```python
from build123d import *

# Parameters (mm, degrees)
SKETCH_1_W                 = 40
SKETCH_1_H                 = 20
EXTRUDE_1_DEPTH            = 28.5
SKETCH_7_R                 = 2.5
EXTRUDE_4_DEPTH            = 6.975384219
SKETCH_1_2_W               = 40
SKETCH_1_2_H               = 20
EXTRUDE_5_DEPTH            = 7.5
SKETCH_3_W                 = 53
SKETCH_3_H                 = 18
EXTRUDE_6_DEPTH            = 2
CUT_EXTRUDE_4_DEPTH        = 5
EXTRUDE_7_DEPTH            = 1.5
SKETCH_13_W                = 12
SKETCH_13_H                = 19
EXTRUDE_8_DEPTH            = 2
SKETCH_14_R                = 6
EXTRUDE_9_DEPTH            = 1.5
EXTRUDE_10_DEPTH           = 0.25
CUT_EXTRUDE_5_DEPTH        = 50
CUT_EXTRUDE_6_DEPTH        = 50
CUT_EXTRUDE_11_DEPTH       = 1.2
SKETCH_25_R                = 1.5
EXTRUDE_12_DEPTH           = 1
EXTRUDE_12_DRAFT           = 15
EXTRUDE_12_PROFILE_2_DEPTH = 1
EXTRUDE_12_PROFILE_2_DRAFT = 15
EXTRUDE_12_PROFILE_3_DEPTH = 1
EXTRUDE_12_PROFILE_3_DRAFT = 15
EXTRUDE_12_PROFILE_4_DEPTH = 1
EXTRUDE_12_PROFILE_4_DRAFT = 15
SKETCH_29_R                = 6.25
EXTRUDE_15_DEPTH           = 1.2
SKETCH_30_R                = 5
EXTRUDE_16_DEPTH           = 0.3
EXTRUDE_17_DEPTH           = 3.5
SKETCH_33_R                = 1.25
CUT_EXTRUDE_12_DEPTH       = 10
FILLET_1_R                 = 2
FILLET_2_R                 = 1
FILLET_4_R                 = 0.5
SKETCH_34_W                = 7
SKETCH_34_H                = 4.5
EXTRUDE_18_DEPTH           = 1
EXTRUDE_19_DEPTH           = 4
EXTRUDE_19_TAPER           = 10


with BuildPart() as part:
    # 草图1 → 凸台-拉伸1 (new body)
    with BuildSketch(Plane(origin=(0, 0, 0), x_dir=(1, 0, 0), z_dir=(0, 1, 0))):
        with Locations((20, -10)):
            Rectangle(SKETCH_1_W, SKETCH_1_H)
    extrude(amount=EXTRUDE_1_DEPTH)

    # 草图7 → 凸台-拉伸4 (add)
    with BuildSketch(Plane(origin=(0, 0, 0), x_dir=(1, 0, 0), z_dir=(0, 1, 0))):
        with Locations(Location((10, -10, 0), (0, 0, 270))):
            Circle(SKETCH_7_R)
    extrude(amount=-EXTRUDE_4_DEPTH)

    # 草图1<2> → 凸台-拉伸5 (add)
    with BuildSketch(Plane(origin=(0, 0, 0), x_dir=(1, 0, 0), z_dir=(0, 1, 0))):
        with Locations((20, -10)):
            Rectangle(SKETCH_1_2_W, SKETCH_1_2_H)
    extrude(amount=-EXTRUDE_5_DEPTH)

    # 草图3 → 凸台-拉伸6 (add)
    with BuildSketch(Plane(origin=(0, 0, 0), x_dir=(1, 0, 0), z_dir=(0, 1, 0))):
        with Locations((20, -10)):
            Rectangle(SKETCH_3_W, SKETCH_3_H)
    extrude(amount=-EXTRUDE_6_DEPTH)

    # 草图8 → 切除-拉伸4 (cut, symmetric)
    with BuildSketch(Plane(origin=(0, 0, 0), x_dir=(1, 0, 0), z_dir=(0, 1, 0))):
        with BuildLine():
            Line((-9.5, -4), (-9.5, -6))
            Line((-9.5, -6), (-6.232050808, -6))
            ThreePointArc((-6.232050808, -6), (-2.5, -5), (-6.232050808, -4))
            Line((-6.232050808, -4), (-9.5, -4))
        make_face()
        with BuildLine():
            Line((-6.232050808, -14), (-9.5, -14))
            Line((-9.5, -14), (-9.5, -16))
            Line((-9.5, -16), (-6.232050808, -16))
            ThreePointArc((-6.232050808, -16), (-2.5, -15), (-6.232050808, -14))
        make_face()
        with BuildLine():
            Line((49.5, -6), (49.5, -4))
            Line((49.5, -4), (46.232050808, -4))
            ThreePointArc((46.232050808, -4), (42.5, -5), (46.232050808, -6))
            Line((46.232050808, -6), (49.5, -6))
        make_face()
        with BuildLine():
            Line((49.5, -16), (49.5, -14))
            Line((49.5, -14), (46.232050808, -14))
            ThreePointArc((46.232050808, -14), (42.5, -15), (46.232050808, -16))
            Line((46.232050808, -16), (49.5, -16))
        make_face()
    extrude(amount=CUT_EXTRUDE_4_DEPTH, both=True, mode=Mode.SUBTRACT)

    # 草图9 → 凸台-拉伸7 (add)
    with BuildSketch(Plane.XZ.offset(7.5)):
        with BuildLine():
            Line((34, 19.5), (34, 0.5))
            Line((34, 0.5), (13.122498999, 0.5))
            ThreePointArc((13.122498999, 0.5), (0, 10), (13.122498999, 19.5))
            Line((13.122498999, 19.5), (34, 19.5))
        make_face()
    extrude(amount=EXTRUDE_7_DEPTH)

    # 草图13 → 凸台-拉伸8 (add)
    with BuildSketch(Plane.XZ.offset(7.5)):
        with Locations((28, 10)):
            Rectangle(SKETCH_13_W, SKETCH_13_H)
    extrude(amount=EXTRUDE_8_DEPTH)

    # 草图14 → 凸台-拉伸9 (add)
    with BuildSketch(Plane.XZ.offset(7.5)):
        with Locations((31, 10)):
            Circle(SKETCH_14_R)
    extrude(amount=EXTRUDE_9_DEPTH)

    # 草图15 → 凸台-拉伸10 (add, symmetric)
    with BuildSketch(Plane(origin=(0, 0, 10), x_dir=(-1, 0, 0), z_dir=(0, 0, -1))):
        Polygon((0, -3.2), (-40, -3.2), (-46.5, -2), (6.5, -2), align=None)
    extrude(amount=EXTRUDE_10_DEPTH, both=True)

    # 草图16 → 切除-拉伸5 (cut, symmetric)
    with BuildSketch(Plane.XY):
        Polygon((0, 26.5), (1.154700538, 28.5), (38.845299462, 28.5), (40, 26.5), (45, 26.5), (45, 36.5), (-5, 36.5), (-5, 26.5), align=None)
    extrude(amount=CUT_EXTRUDE_5_DEPTH, both=True, mode=Mode.SUBTRACT)

    # 草图18 → 切除-拉伸6 (cut, symmetric)
    with BuildSketch(Plane(origin=(0, 0, 0), x_dir=(0, 0, -1), z_dir=(1, 0, 0))):
        Polygon((-20, 26.5), (-18.845299462, 28.5), (-1.154700538, 28.5), (0, 26.5), (15, 26.5), (15, 36.5), (-35, 36.5), (-35, 26.5), align=None)
    extrude(amount=CUT_EXTRUDE_6_DEPTH, both=True, mode=Mode.SUBTRACT)

    # 草图22 → 切除-拉伸11 (cut)
    with BuildSketch(Plane(origin=(0, 28.5, 0), x_dir=(1, 0, 0), z_dir=(0, 1, 0))):
        with BuildLine():
            ThreePointArc((1.5, -3.5), (2.914213562, -2.914213562), (3.5, -1.5))
            Line((3.5, -1.5), (3.5, 0.5))
            Line((3.5, 0.5), (-0.5, 0.5))
            Line((-0.5, 0.5), (-0.5, -3.5))
            Line((-0.5, -3.5), (1.5, -3.5))
        make_face()
        with BuildLine():
            Line((3.5, -20.5), (3.5, -18.5))
            ThreePointArc((3.5, -18.5), (2.914213562, -17.085786438), (1.5, -16.5))
            Line((1.5, -16.5), (-0.5, -16.5))
            Line((-0.5, -16.5), (-0.5, -20.5))
            Line((-0.5, -20.5), (3.5, -20.5))
        make_face()
        with BuildLine():
            ThreePointArc((38.5, -16.5), (37.085786438, -17.085786438), (36.5, -18.5))
            Line((36.5, -18.5), (36.5, -20.5))
            Line((36.5, -20.5), (40.5, -20.5))
            Line((40.5, -20.5), (40.5, -16.5))
            Line((40.5, -16.5), (38.5, -16.5))
        make_face()
        with BuildLine():
            Line((36.5, 0.5), (36.5, -1.5))
            ThreePointArc((36.5, -1.5), (37.085786438, -2.914213562), (38.5, -3.5))
            Line((38.5, -3.5), (40.5, -3.5))
            Line((40.5, -3.5), (40.5, 0.5))
            Line((40.5, 0.5), (36.5, 0.5))
        make_face()
    extrude(amount=-CUT_EXTRUDE_11_DEPTH, mode=Mode.SUBTRACT)


with BuildPart() as extrude_12_tool:
    # 草图25 → 凸台-拉伸12 (with draft: the straight prism first)
    with BuildSketch(Plane(origin=(0, 27.3, 0), x_dir=(1, 0, 0), z_dir=(0, 1, 0))):
        with Locations((1.5, -1.5)):
            Circle(SKETCH_25_R)
    extrude(amount=EXTRUDE_12_DEPTH)
    # 凸台-拉伸12: the draft: its side faces are tilted about the plane it starts from
    extrude_12_sides = [extrude_12_tool.faces().sort_by_distance(p)[0] for p in [
        (0, 27.8, 1.5),
    ]]
    draft(extrude_12_sides, Plane(origin=(0, 27.3, 0), x_dir=(1, 0, 0), z_dir=(0, 1, 0)), EXTRUDE_12_DRAFT)


with BuildPart() as part_1:
    add(part.part)

    # 凸台-拉伸12: add extrude_12_tool
    add(extrude_12_tool.part)


with BuildPart() as extrude_12_profile_2_tool:
    # 草图25 → 凸台-拉伸12 profile 2 (with draft: the straight prism first)
    with BuildSketch(Plane(origin=(0, 27.3, 0), x_dir=(1, 0, 0), z_dir=(0, 1, 0))):
        with Locations((38.5, -1.5)):
            Circle(SKETCH_25_R)
    extrude(amount=EXTRUDE_12_PROFILE_2_DEPTH)
    # 凸台-拉伸12 profile 2: the draft: its side faces are tilted about the plane it starts from
    extrude_12_profile_2_sides = [extrude_12_profile_2_tool.faces().sort_by_distance(p)[0] for p in [
        (37, 27.8, 1.5),
    ]]
    draft(extrude_12_profile_2_sides, Plane(origin=(0, 27.3, 0), x_dir=(1, 0, 0), z_dir=(0, 1, 0)), EXTRUDE_12_PROFILE_2_DRAFT)


with BuildPart() as part_2:
    add(part_1.part)

    # 凸台-拉伸12 profile 2: add extrude_12_profile_2_tool
    add(extrude_12_profile_2_tool.part)


with BuildPart() as extrude_12_profile_3_tool:
    # 草图25 → 凸台-拉伸12 profile 3 (with draft: the straight prism first)
    with BuildSketch(Plane(origin=(0, 27.3, 0), x_dir=(1, 0, 0), z_dir=(0, 1, 0))):
        with Locations((38.5, -18.5)):
            Circle(SKETCH_25_R)
    extrude(amount=EXTRUDE_12_PROFILE_3_DEPTH)
    # 凸台-拉伸12 profile 3: the draft: its side faces are tilted about the plane it starts from
    extrude_12_profile_3_sides = [extrude_12_profile_3_tool.faces().sort_by_distance(p)[0] for p in [
        (37, 27.8, 18.5),
    ]]
    draft(extrude_12_profile_3_sides, Plane(origin=(0, 27.3, 0), x_dir=(1, 0, 0), z_dir=(0, 1, 0)), EXTRUDE_12_PROFILE_3_DRAFT)


with BuildPart() as part_3:
    add(part_2.part)

    # 凸台-拉伸12 profile 3: add extrude_12_profile_3_tool
    add(extrude_12_profile_3_tool.part)


with BuildPart() as extrude_12_profile_4_tool:
    # 草图25 → 凸台-拉伸12 profile 4 (with draft: the straight prism first)
    with BuildSketch(Plane(origin=(0, 27.3, 0), x_dir=(1, 0, 0), z_dir=(0, 1, 0))):
        with Locations((1.5, -18.5)):
            Circle(SKETCH_25_R)
    extrude(amount=EXTRUDE_12_PROFILE_4_DEPTH)
    # 凸台-拉伸12 profile 4: the draft: its side faces are tilted about the plane it starts from
    extrude_12_profile_4_sides = [extrude_12_profile_4_tool.faces().sort_by_distance(p)[0] for p in [
        (0, 27.8, 18.5),
    ]]
    draft(extrude_12_profile_4_sides, Plane(origin=(0, 27.3, 0), x_dir=(1, 0, 0), z_dir=(0, 1, 0)), EXTRUDE_12_PROFILE_4_DRAFT)


with BuildPart() as part_4:
    add(part_3.part)

    # 凸台-拉伸12 profile 4: add extrude_12_profile_4_tool
    add(extrude_12_profile_4_tool.part)

    # 草图29 → 凸台-拉伸15 (add)
    with BuildSketch(Plane.XZ.offset(9)):
        with Locations(Location((10, 10, 0), (0, 0, 270))):
            Circle(SKETCH_29_R)
    extrude(amount=EXTRUDE_15_DEPTH)

    # 草图30 → 凸台-拉伸16 (add)
    with BuildSketch(Plane.XZ.offset(10.2)):
        with Locations(Location((10, 10, 0), (0, 0, 270))):
            Circle(SKETCH_30_R)
    extrude(amount=EXTRUDE_16_DEPTH)

    # 草图31 → 凸台-拉伸17 (add)
    with BuildSketch(Plane.XZ.offset(10.5)):
        Polygon((12.976344104, 10.375999701), (12.421457903, 10.621724718), (12.789329458, 11.104373658), (12.1907667, 11.204384185), (12.427050983, 11.763355757), (11.822421569, 11.711367765), (11.912271969, 12.311539728), (11.339566987, 12.110819814), (11.277337875, 12.714481157), (10.772542486, 12.377641291), (10.562143944, 12.946861752), (10.156976299, 12.495066821), (9.811628441, 12.994080185), (9.531546714, 12.455718127), (9.072949017, 12.853169549), (8.935551771, 12.262067631), (8.392519615, 12.532983777), (8.406440026, 11.926283107), (7.813094118, 12.053641318), (7.977457514, 11.469463131), (7.37107996, 11.445261022), (7.675558785, 10.920311382), (7.094250517, 10.746069661), (7.519713247, 10.313333084), (7, 10), (7.519713247, 9.686666916), (7.094250517, 9.253930339), (7.675558785, 9.079688618), (7.37107996, 8.554738978), (7.977457514, 8.530536869), (7.813094118, 7.946358682), (8.406440026, 8.073716893), (8.392519615, 7.467016223), (8.935551771, 7.737932369), (9.072949017, 7.146830451), (9.531546714, 7.544281873), (9.811628441, 7.005919815), (10.156976299, 7.504933179), (10.562143944, 7.053138248), (10.772542486, 7.622358709), (11.277337875, 7.285518843), (11.339566987, 7.889180186), (11.912271969, 7.688460272), (11.822421569, 8.288632235), (12.427050983, 8.236644243), (12.1907667, 8.795615815), (12.789329458, 8.895626342), (12.421457903, 9.378275282), (12.976344104, 9.624000299), (12.5, 10), align=None)
    extrude(amount=EXTRUDE_17_DEPTH)

    # 草图33 → 切除-拉伸12 (cut)
    with BuildSketch(Plane.XZ.offset(10.5)):
        with Locations(Location((10, 10, 0), (0, 0, 90))):
            Circle(SKETCH_33_R)
    extrude(amount=CUT_EXTRUDE_12_DEPTH, mode=Mode.SUBTRACT)

    # 圆角1
    fillet_1_edges = [part_4.edges().sort_by_distance(p)[0] for p in [
        (-6.5, -1, 1),
        (46.5, -1, 19),
        (-6.5, -1, 19),
        (46.5, -1, 1),
    ]]
    fillet(fillet_1_edges, radius=FILLET_1_R)

    # 圆角2
    fillet_2_edges = [part_4.edges().sort_by_distance(p)[0] for p in [
        (40, 9.5, 0),
        (0, 9.5, 0),
        (0, 9.5, 20),
        (40, 9.5, 20),
    ]]
    fillet(fillet_2_edges, radius=FILLET_2_R - 0.0001)  # a hair under: the kernel refuses the full size

    # 圆角4
    fillet_4_edges = [part_4.edges().sort_by_distance(p)[0] for p in [
        (0.267949192, 28.3, 1.5),
        (37.267949192, 28.3, 1.5),
        (37.267949192, 28.3, 18.5),
        (0.267949192, 28.3, 18.5),
    ]]
    fillet(fillet_4_edges, radius=FILLET_4_R)

    # 草图34 → 凸台-拉伸18 (add)
    with BuildSketch(Plane.ZY):
        with Locations((10, 21.5)):
            Rectangle(SKETCH_34_W, SKETCH_34_H)
    extrude(amount=EXTRUDE_18_DEPTH)

    # 草图35 → 凸台-拉伸19 (add)
    with BuildSketch(Plane.ZY.offset(1)):
        with BuildLine():
            ThreePointArc((8.5, 23.5), (6.5, 21.5), (8.5, 19.5))
            Line((8.5, 19.5), (11.5, 19.5))
            ThreePointArc((11.5, 19.5), (13.5, 21.5), (11.5, 23.5))
            Line((11.5, 23.5), (8.5, 23.5))
        make_face()
    extrude(amount=EXTRUDE_19_DEPTH, taper=EXTRUDE_19_TAPER)


solid = part_4.part
```
Build history of the part. All positions in model axes, mm. A direction names the side the tool comes from. Round coordinates to 2 decimals unless told otherwise and drop trailing zeros. Write each loop counter-clockwise with the first axis right and the second up, starting at its lowest first coordinate (ties: lowest second). Pieces come first, ordered by that corner, then holes. Notation, with made-up numbers: (76, 21) -> (120, 21) arc R32 ccw to (120, 55) -> close; hole circle Ø11 at (-0.5, -32). An arc over 180 degrees is marked (long way). Put each result on its own line as item: value.
Item 1: Flat gauge pins, fed straight in: P1, Ø0.5, axis at x = 1.5, z = 18.5, coming from the +Y side; P2, Ø2, axis at x = 39, z = 19.5, coming from the -Y side; P3, Ø8, axis at x = 24, y = -8, coming from the -Z side; P4, Ø5, axis at y = 13.5, z = 10.5, coming from the -X side. Where does each tip first touch, or does it go through?
Here are the results:
P1: stops at y = 28.3
P2: stops at y = -7.5
P3: stops at z = 0
P4: stops at x = 0
Item 2: Wall check: probe 1 along Z at (x, y) = (10, -12.3); probe 2 along Z at (x, y) = (44, -1); probe 3 along Y at (x, z) = (17.5, 5). Give the ranges that are in metal, low to high. Write a range as from..to.
Here are the results:
probe 1: z = 7.28..8.75, 11.25..12.72
probe 2: z = 1..3.06, 6.94..13.06, 16.94..19
probe 3: y = -9..28.5
Item 3: Tool access for faces 5 (the face through (6.2, -9.59, 14.96)), 6 (the face through (-5, 21, 10)), 7 (the face through (2, -7.5, 18)), 8 (the face through (38.5, 28.3, 18.5)), 9 (the face through (2.93, 27.91, 17.1)): list every direction of +Z, -Z, +X, -X, +Y, -Y with a clear straight run to the whole face (end or side of a thin tool).
Here are the results:
face 5: -Y
face 6: +Z, -Z, -X, +Y
face 7: +Z, -X, -Y
face 8: +Z, +X, +Y
face 9: +Y
Item 4: Slice it at B-B, the plane y = 16. Give the cut face in (x, z), plus the area to 3 significant figures.
Here are the results:
outline: (0, 1) arc R1 ccw to (1, 0) -> (39, 0) arc R1 ccw to (40, 1) -> (40, 19) arc R1 ccw to (39, 20) -> (1, 20) arc R1 ccw to (0, 19) -> close
area: 799 mm^2
Item 5: Slice it at A-A, the plane x = 18.5. Give the cut face in (y, z), plus the area to 3 significant figures.
Here are the results:
outline: (-9, 0.5) -> (-7.5, 0.5) -> (-7.5, 0) -> (26.5, 0) -> (28.5, 1.15) -> (28.5, 18.85) -> (26.5, 20) -> (-7.5, 20) -> (-7.5, 19.5) -> (-9, 19.5) -> close
area: 746 mm^2
Item 6: Two-plate mould, pull along Z, no slides. Class faces 1 (the face through (37.1, 27.91, 17.07)), 2 (the face through (0.57, 27.49, 10.14)), 3 (the face through (42, -1, 1)), 4 (the face through (-2.6, -2, 13.6)): pulls with the +Z half, pulls with the -Z half, needs draft (parallel to the pull), parting line crosses it, or undercut.
Here are the results:
face 1: undercut
face 2: undercut
face 3: pulls with the -Z half
face 4: needs draft
Item 7: Slice it at C-C, the plane x = 35.5. Give the cut face in (y, z), plus the area to 3 significant figures.
Here are the results:
outline: (-9, 6.03) -> (-7.5, 6.03) -> (-7.5, 0) -> (26.5, 0) -> (28.5, 1.15) -> (28.5, 18.85) -> (26.5, 20) -> (-7.5, 20) -> (-7.5, 13.97) -> (-9, 13.97) -> close
area: 730 mm^2
